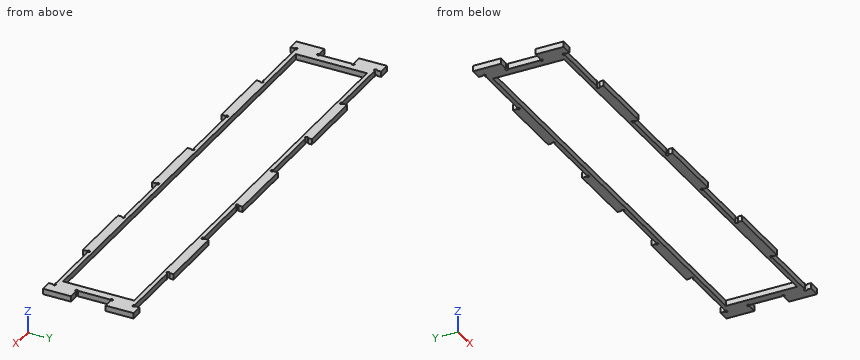
Autodesk Inventor part; units mm, degrees
ref_plane "YZ Plane" through (0, 0, 0) normal (1, 0, 0) x (0, 1, 0)
ref_plane "XZ Plane" through (0, 0, 0) normal (0, 1, 0) x (-1, 0, 0)
ref_plane "XY Plane" through (0, 0, 0) normal (0, 0, 1) x (1, 0, 0)
sketch "Sketch1" plane through (0, 0, 0) normal (0, 0, 1) x (1, 0, 0)
  line L0 (-173, 32.5) -> (173, 32.5)
  line L1 (173, 32.5) -> (173, -32.5)
  line L2 (173, -32.5) -> (-173, -32.5)
  line L3 (-173, -32.5) -> (-173, 32.5)
  point P0 (0, 0)
  point P1 (173, 0)
  point P2 (0, 32.5)
  dimension "d0" = 65
  dimension "d1" = 346
extrude "Extrusion1" add sketch "Sketch1" along normal blind 4
sketch "Sketch2" plane through (0, 0, 4) normal (0, 0, 1) x (1, 0, 0)
  line L0 (-159, 25.5) -> (159, 25.5)
  line L1 (159, 25.5) -> (159, -25.5)
  line L2 (159, -25.5) -> (-159, -25.5)
  line L3 (-159, -25.5) -> (-159, 25.5)
  line L4 (173, 32.5) -> (-173, 32.5)
  line L5 (-173, 32.5) -> (-173, -32.5)
  line L6 (-173, -32.5) -> (173, -32.5)
  line L7 (173, -32.5) -> (173, 32.5)
  point P0 (0, 0)
  dimension "d4" = 7
  dimension "d5" = 14
  dimension "d6" = 7
  dimension "d7" = 14
extrude "Extrusion2" cut sketch "Sketch2" against normal blind 10 contours L0 L1 L2 L3
sketch "Esboço3" plane through (0, 0, 4) normal (0, 0, 1) x (1, 0, 0)
  line L0 (-118.5, 32.5) -> (-118.5, 28.5)
  line L1 (-118.5, 28.5) -> (-165, 28.5)
  line L2 (-70.5, 32.5) -> (-24, 32.5)
  line L3 (-24, 32.5) -> (-24, 28.5)
  line L4 (-24, 28.5) -> (-70.5, 28.5)
  line L5 (-70.5, 28.5) -> (-70.5, 32.5)
  circle A0 centre (-118.5, 28.5) radius 1
  circle A1 centre (-70.5, 28.5) radius 1
  circle A2 centre (-24, 28.5) radius 1
  line L6 (-165, 28.5) -> (-165, 32.5)
  line L7 (-165, 32.5) -> (-118.5, 32.5)
  line L8 (173, 32.5) -> (-173, 32.5)
  line L9 (-173, 32.5) -> (-173, -32.5)
  circle A3 centre (-165, 28.5) radius 1
  point P0 (0, 0)
  dimension "d12" = 46.5
  dimension "d13" = 48
  dimension "d14" = 2
  dimension "d15" = 2
  dimension "d16" = 2
  dimension "d19" = 8
  dimension "d20" = 46.5
  dimension "d21" = 2
extrude "Extrusão3" cut sketch "Esboço3" against normal blind 10
mirror "Espelhamento1" about plane through (0, 0, 0) normal (1, 0, 0) of "Extrusão3"
mirror "Espelhamento2" about plane through (0, 0, 0) normal (0, 1, 0) of "Extrusão3", "Espelhamento1"
sketch "Esboço4" plane through (0, 0, 4) normal (0, 0, 1) x (1, 0, 0)
  line L0 (-173, 32.5) -> (-173, -32.5)
  line L1 (-173, -12.5) -> (-165, -12.5)
  line L2 (-165, -12.5) -> (-165, 12.5)
  line L3 (-165, 12.5) -> (-173, 12.5)
  line L4 (-173, 12.5) -> (-173, -12.5)
  line L5 (-165, 32.5) -> (-173, 32.5)
  line L6 (-173, -32.5) -> (-165, -32.5)
  circle A0 centre (-165, 12.5) radius 1
  circle A1 centre (-165, -12.5) radius 1
  point P0 (0, 0)
  dimension "d22" = 8
  dimension "d23" = 20
  dimension "d24" = 25
  dimension "d25" = 20
  dimension "d26" = 2
  dimension "d27" = 2
extrude "Extrusão4" cut sketch "Esboço4" against normal blind 10
mirror "Espelhamento3" about plane through (0, 0, 0) normal (1, 0, 0) of "Extrusão4"
properties part number "letreiro"
Work out the finished part from the listing and answer in its coordinate system (mm). Give positions to 0.01 mm unless a question says otherwise; leave off trailing zeros. Loops run counter-clockwise (first coordinate to the right, second up) from the corner with the lowest first, then second, coordinate; pieces in that order, holes last. Notation, with made-up numbers: (22.25, 37) -> (41.25, 37) arc R24 cw to (41.25, 47) -> close; hole circle Ø4 at (18.25, 40). An arc over 180 degrees is marked (long way). One line per question, with ' | ' between items. Start each with the question number.
1) Section A-A, the plane x = 3 is taken. Determine the outline of the cut face in (y, z), then the cut area to 3 significant figures.
2) Section B-B, the plane y = -7 is taken. Determine the outline of the cut face in (x, z), then the cut area to 3 significant figures.
3) Each of these flat-tipped pins is pushed along its axis until it touches: pin 1 (1 mm diameter, centred on y = -1.5, z = 1, fed in from +X); pin 2 (1.5 mm diameter, centred on x = -69.5, z = 1, fed in from -Y); pin 3 (1.2 mm diameter, centred on x = 51.5, z = 1, fed in from +Y). Where does it stop, or does it pass through?
4) Straight lines are drawn through the part: L1, parallel to Y at x = 69, z = 0.85; L2, parallel to Y at x = -19, z = 1.5; L3, parallel to X at y = -6.5, z = 1.3. For each, find the intervals that lie inside material, in ascending order.
Resolved:
1) outline: (-32.5, 0) -> (-25.5, 0) -> (-25.5, 4) -> (-32.5, 4) -> close; (25.5, 0) -> (32.5, 0) -> (32.5, 4) -> (25.5, 4) -> close | area: 56.0 mm2
2) outline: (-165, 0) -> (-159, 0) -> (-159, 4) -> (-165, 4) -> close; (159, 0) -> (165, 0) -> (165, 4) -> (159, 4) -> close | area: 48.0 mm2
3) pin 1: x = 165 | pin 2: y = -28.5 | pin 3: y = 28.5
4) L1: -28.5 to -25.5, 25.5 to 28.5 | L2: -32.5 to -25.5, 25.5 to 32.5 | L3: -165 to -159, 159 to 165
